Design review of the part shown in the three views and the two pictorial views. Dimensions are in mm from the part's minimum x, y and z. A direction names the side the tool comes from. Round coordinates to 2 decimals unless told otherwise and drop trailing zeros. Order: outer loops, then holes, each group sorted by start corner. A loop starts at its lowest first (then second) coordinate and runs counter-clockwise, first axis right, second up.
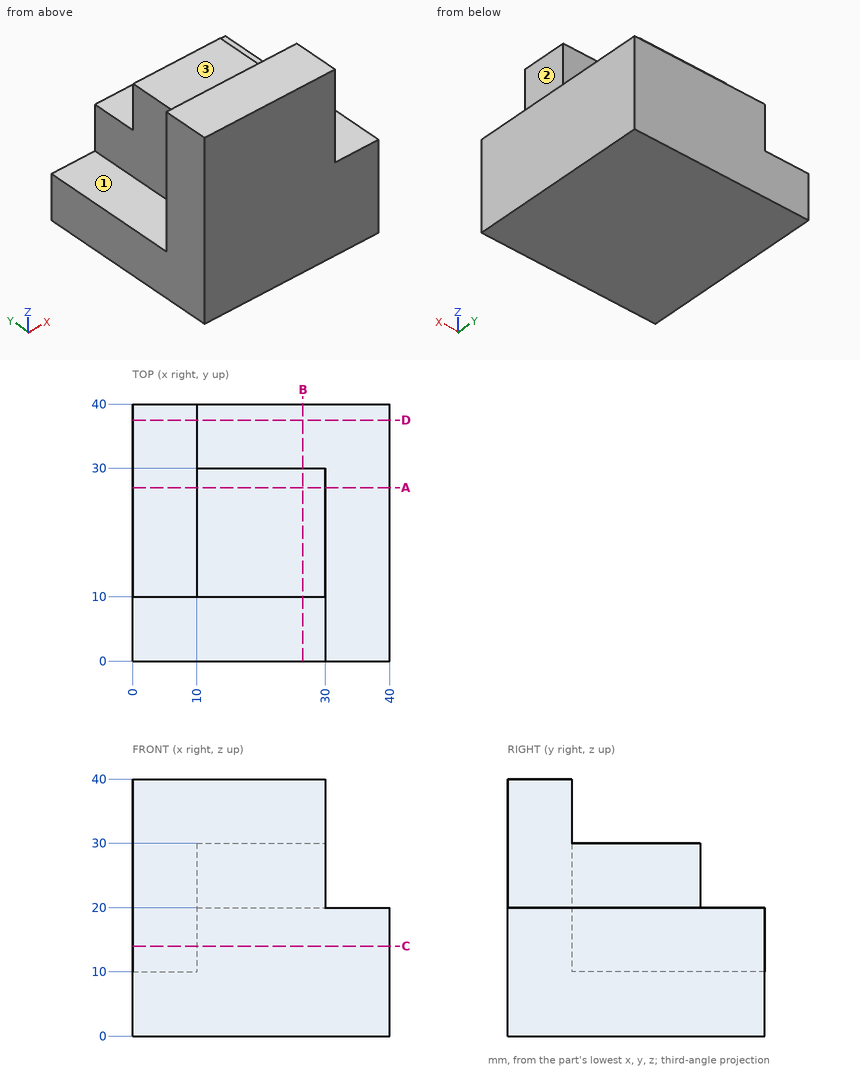
(1) Add section C-C on z = 14. Give the boundary of the cut face in (x, y), plus the area to 3 significant figures.
(2) Add section B-B on x = 26.5. Give the boundary of the cut face in (y, z).
(3) Add section A-A on y = 27. Give the boundary of the cut face in (x, z).
(4) Wall thickness on L1, parallel to Z at x = 18.5, y = 10.5; L2, parallel to Z at x = 7.5, y = 34.5: over which ranges is each line inside the solid? List them lowest first.
(5) Add section D-D on y = 37.5. Give the boundary of the cut face in (x, z).
(6) Clearance check with flat-ended pins moving along their axes: P1, Ø4, axis at x = 22.5, y = 26.5, coming from the +Z side; P2, Ø3, axis at x = 27, y = 32.5, coming from the +Z side; P3, Ø16, axis at y = 17.5, z = 34.5, coming from the +X side. State where each tip first meets the part, or that it passes through.
(7) Tool access review of the marked faces 1, 2 and 3: name each direction out of +Z, -Z, +X, -X, +Y, -Y from which nothing blocks a thin tool from reaching the whole face with its end or side.
Here are the results:
1. outline: (0, 0) - (40, 0) - (40, 40) - (10, 40) - (10, 10) - (0, 10) - close
1. area: 1,300 mm2
2. outline: (0, 0) - (40, 0) - (40, 20) - (30, 20) - (30, 30) - (10, 30) - (10, 40) - (0, 40) - close
3. outline: (0, 0) - (40, 0) - (40, 20) - (30, 20) - (30, 30) - (10, 30) - (10, 10) - (0, 10) - close
4. L1: z = 0 to 30
4. L2: z = 0 to 10
5. outline: (0, 0) - (40, 0) - (40, 20) - (10, 20) - (10, 10) - (0, 10) - close
6. P1: stops at z = 30
6. P2: stops at z = 20
6. P3: stops at x = 30
7. face 1: +Z, -X, +Y
7. face 2: +Z, +X, +Y, -Y
7. face 3: +Z, +X, -X, +Y
